Here's how the part is built. I have some questions about the finished solid (model axes, mm). Face numbers are marked on the shaded views. Round coordinates to 2 decimals unless told otherwise and drop trailing zeros. Write each loop counter-clockwise with the first axis right and the second up, starting at its lowest first coordinate (ties: lowest second). Pieces come first, ordered by that corner, then holes. Notation, with made-up numbers: (-15.5, 11) - (3.5, 11) arc R5 ccw to (3.5, 15) - close; hole circle Ø9 at (50, -34). An arc over 180 degrees is marked (long way). One line per item, written item: value. Start each with the question number.
Item 1: If I drill on line 1 (X direction, y = 0, z = 10); line 2 (X direction, y = 0, z = 6.5); line 3 (Y direction, x = 10, z = 9.25), over which ranges is the centre line in solid material (lowest first)?
Item 2: Imagine slicing it at B-B, the plane y = 0. Please give me the cut outline in (x, z).
Item 3: Thinking about a two-plate mould opening in Z: for the marked faces 1, 2, 3 and 4, which applies, released by +Z, released by -Z, zero draft, split by the parting line, or undercut?
Item 4: Imagine slicing it at C-C, the plane x = 0. Please give me the cut outline in (y, z).
Item 5: Imagine slicing it at D-D, the plane y = -6.75. Please give me the cut outline in (x, z).
Item 6: Imagine slicing it at A-A, the plane z = 6.5. Please give me the cut outline in (x, y), then the cut area to 3 significant figures.
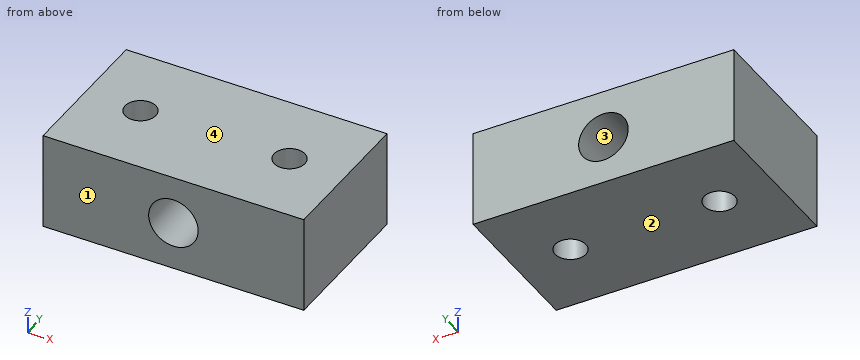
Autodesk Inventor part; units mm, degrees
ref_plane "YZ Plane" through (0, 0, 0) normal (1, 0, 0) x (0, 1, 0)
ref_plane "XZ Plane" through (0, 0, 0) normal (0, 1, 0) x (-1, 0, 0)
ref_plane "XY Plane" through (0, 0, 0) normal (0, 0, 1) x (1, 0, 0)
sketch "Sketch1" plane through (0, 0, 0) normal (0, 0, 1) x (1, 0, 0)
  line L0 (-17.5, 10) -> (17.5, 10)
  line L1 (17.5, 10) -> (17.5, -10)
  line L2 (17.5, -10) -> (-17.5, -10)
  line L3 (-17.5, -10) -> (-17.5, 10)
  point P0 (0, 0)
  dimension "d0" = 35
  dimension "d1" = 20
  dimension "d2" = 10
  dimension "d3" = 17.5
extrude "Extrusion1" add sketch "Sketch1" along normal blind 13
sketch "Sketch2" plane through (0, 0, 13) normal (0, 0, 1) x (1, 0, 0)
  line L0 (-17.5, 10) -> (17.5, 10)
  line L1 (-17.5, -10) -> (-17.5, 10)
  circle A0 centre (-10, 0) radius 2.1
  circle A1 centre (10, 0) radius 2.1
  point P0 (0, 0)
  dimension "d6" = 4.2
  dimension "d7" = 4.2
  dimension "d8" = 20
  dimension "d9" = 10
  dimension "d10" = 10
  dimension "d11" = 7.5
hole "Hole1" at (-10, 0, 13) at (10, 0, 13) direction (0, 0, -1) diameter 4.134 end through all
sketch "Sketch3" plane through (-17.5, 10, 0) normal (0, 1, 0) x (1, 0, 0)
  line L0 (0, 0) -> (35, 0)
  line L1 (0, 0) -> (0, -13)
  circle A0 centre (17.5, -6.5) radius 3.375
  point P0 (17.5, 0)
  dimension "d19" = 6.75
  dimension "d20" = 17.5
  dimension "d21" = 6.5
hole "Hole2" at (0, 10, 6.5) direction (0, -1, 0) diameter 6.647 end through all
properties part number "PS20010" material "Acetal Resin, Black"
Values follow:
1. line 1: x = -17.5 to -12.07, -7.93 to 7.93, 12.07 to 17.5
1. line 2: x = -17.5 to -12.07, -7.93 to -3.32, 3.32 to 7.93, 12.07 to 17.5
1. line 3: y = -10 to -2.07, 2.07 to 10
2. outline: (-17.5, 0) - (-12.07, 0) - (-12.07, 13) - (-17.5, 13) - close; (-7.93, 0) - (7.93, 0) - (7.93, 13) - (-7.93, 13) - close; (12.07, 0) - (17.5, 0) - (17.5, 13) - (12.07, 13) - close; hole circle Ø6.65 at (0, 6.5)
3. face 1: zero draft
3. face 2: released by -Z
3. face 3: undercut
3. face 4: released by +Z
4. outline: (-10, 0) - (10, 0) - (10, 3.18) - (-10, 3.18) - close; (-10, 9.82) - (10, 9.82) - (10, 13) - (-10, 13) - close
5. outline: (-17.5, 0) - (17.5, 0) - (17.5, 13) - (-17.5, 13) - close; hole circle Ø6.65 at (0, 6.5)
6. outline: (-17.5, -10) - (-3.32, -10) - (-3.32, 10) - (-17.5, 10) - close; (3.32, -10) - (17.5, -10) - (17.5, 10) - (3.32, 10) - close; hole circle Ø4.13 at (-10, 0); hole circle Ø4.13 at (10, 0)
6. area: 540 mm^2
